from build123d import *

# Parameters (mm, degrees)
SKETCH2_W           = 32.5
SKETCH2_H           = 32.5
SKETCH2_R           = 1
BOSS_EXTRUDE1_DEPTH = 1.5
SKETCH4_W           = 13
SKETCH4_H           = 13
BOSS_EXTRUDE2_DEPTH = 4
SKETCH6_W           = 10
SKETCH6_H           = 4.75
BOSS_EXTRUDE3_DEPTH = 6


with BuildPart() as part:
    # Sketch2 → Boss-Extrude1 (new body)
    with BuildSketch(Plane.XY):
        Rectangle(SKETCH2_W, SKETCH2_H)
        with Locations((13.875, 13.875)):
            Circle(SKETCH2_R, mode=Mode.SUBTRACT)
        with Locations((13.875, -13.875)):
            Circle(SKETCH2_R, mode=Mode.SUBTRACT)
        with Locations((-13.875, -13.875)):
            Circle(SKETCH2_R, mode=Mode.SUBTRACT)
        with Locations((-13.875, 13.875)):
            Circle(SKETCH2_R, mode=Mode.SUBTRACT)
    extrude(amount=BOSS_EXTRUDE1_DEPTH)

    # Sketch4 → Boss-Extrude2 (add)
    with BuildSketch(Plane.XY.offset(1.5)):
        Rectangle(SKETCH4_W, SKETCH4_H)
        with BuildLine():
            Line((8.925, -1.85), (-8.925, -1.85))
            ThreePointArc((-8.925, -1.85), (-10.775, 0), (-8.925, 1.85))
            Line((-8.925, 1.85), (8.925, 1.85))
            ThreePointArc((8.925, 1.85), (10.775, 0), (8.925, -1.85))
        make_face()
    extrude(amount=BOSS_EXTRUDE2_DEPTH)

    # Sketch5 → Revolve1 (revolve)
    with BuildSketch(Plane(origin=(0, 0, 0), x_dir=(1, 0, 0), z_dir=(0, 1, 0)), mode=Mode.PRIVATE) as revolve1_sk:
        Polygon((0, -5.5), (6.5, -5.5), (6.5, -13.4), (5.65, -13.4), (5.65, -18.4), (8.5, -18.4), (8.5, -22.9), (0, -22.9), align=None)
    revolve(revolve1_sk.sketch.rotate(Axis((0, 0, 0), (0, 0, 1)), 180), axis=Axis((0, 0, 0), (0, 0, 1)))

    # Sketch6 → Boss-Extrude3 (add)
    with BuildSketch(Plane(origin=(0, 0, 0), x_dir=(-1, 0, 0), z_dir=(0, 0, -1))):
        with Locations((0, -13.875)):
            Rectangle(SKETCH6_W, SKETCH6_H)
    extrude(amount=BOSS_EXTRUDE3_DEPTH)


solid = part.part
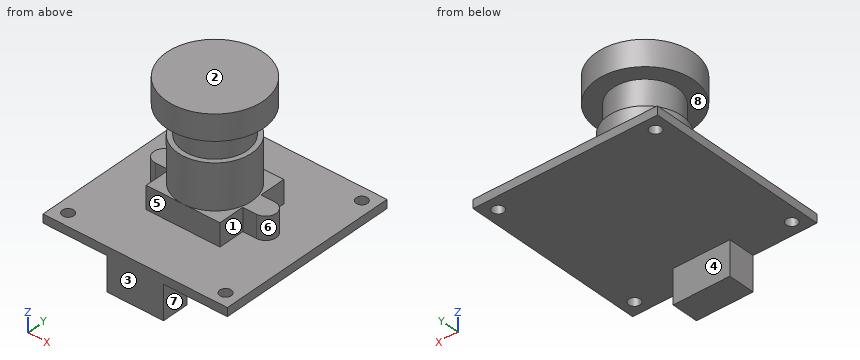
Can you work these out from the model? Positions are in its coordinate system, mm. Face numbers are marked on the shaded views. A direction names the side the tool comes from. Give positions to 0.01 mm unless a question says otherwise; leave off trailing zeros. Loops run counter-clockwise (first coordinate to the right, second up) from the corner with the lowest first, then second, coordinate; pieces in that order, holes last. Notation, with made-up numbers: (53, 80.25) - (92, 80.25) arc R18 ccw to (92, 90.25) - close; hole circle Ø8 at (12, 36.5). An arc over 180 degrees is marked (long way). Return JSON: item names as keys, results as strings.
1. We'd pull the mould along Z, two halves only. Please class the marked faces 1, 2 and 3: +Z half, -Z half, draft (parallel to the pull), parting line (faces both ways), or undercut.
Output values:
{"face 1": "undercut", "face 2": "+Z half", "face 3": "draft"}
2. I want a section at C-C on x = -3. Please give me the cut outline in (y, z).
Output values:
{"outline": "(-16.25, -6) - (-11.5, -6) - (-11.5, 0) - (16.25, 0) - (16.25, 1.5) - (6.5, 1.5) - (6.5, 5.5) - (5.77, 5.5) - (5.77, 13.4) - (4.79, 13.4) - (4.79, 18.4) - (7.95, 18.4) - (7.95, 22.9) - (-7.95, 22.9) - (-7.95, 18.4) - (-4.79, 18.4) - (-4.79, 13.4) - (-5.77, 13.4) - (-5.77, 5.5) - (-6.5, 5.5) - (-6.5, 1.5) - (-16.25, 1.5) - close"}
3. If I drill on line 1 (Z direction, x = 5, y = 6); line 2 (Y direction, x = 0, z = 20); line 3 (Z direction, x = 10, y = -13), over which ranges is the centre line in solid material (lowest first)?
Output values:
{"line 1": "z = 0 to 5.5, 18.4 to 22.9", "line 2": "y = -8.5 to 8.5", "line 3": "z = 0 to 1.5"}
4. I want a section at A-A on y = -12. Please give me the cut outline in (x, z), and give its area (3 significant figures).
Output values:
{"outline": "(-16.25, 0) - (-5, 0) - (-5, -6) - (5, -6) - (5, 0) - (16.25, 0) - (16.25, 1.5) - (-16.25, 1.5) - close", "area": "109 mm²"}
5. I want a section at D-D on y = 0. Please give me the cut outline in (x, z) (3 decimals), and give its area (3 significant figures).
Output values:
{"outline": "(-16.25, 0) - (16.25, 0) - (16.25, 1.5) - (10.775, 1.5) - (10.775, 5.5) - (6.5, 5.5) - (6.5, 13.4) - (5.65, 13.4) - (5.65, 18.4) - (8.5, 18.4) - (8.5, 22.9) - (-8.5, 22.9) - (-8.5, 18.4) - (-5.65, 18.4) - (-5.65, 13.4) - (-6.5, 13.4) - (-6.5, 5.5) - (-10.775, 5.5) - (-10.775, 1.5) - (-16.25, 1.5) - close", "area": "371 mm²"}
6. I want a section at B-B on z = -1.75. Please give me the cut outline in (x, y).
Output values:
{"outline": "(-5, -16.25) - (5, -16.25) - (5, -11.5) - (-5, -11.5) - close"}
7. For the marked faces 4, 5, 6, 7 and 8, which set-ups out of +Z, -Z, +X, -X, +Y, -Y let a thin tool reach every point of the face, with its end or its side?
Output values:
{"face 4": "-Z, +X, -X, +Y", "face 5": "+X, -X, -Y", "face 6": "+Z, +X", "face 7": "-Z, +X, +Y, -Y", "face 8": "none"}
8. I'm going to push flat-ended pins straight in: pin 1 Ø1.2 at (x, y) = (-13.875, 13.875) entering from -Z; pin 2 Ø4 at (x, z) = (7, 18.5) entering from +Y; pin 3 Ø1.9 at (x, z) = (-7, 3) entering from +Y; pin 4 Ø1.2 at (x, z) = (-8.5, 3) entering from -Y. Where does each tip first touch, or does it pass through?
Output values:
{"pin 1": "passes through", "pin 2": "stops at y = 6.87", "pin 3": "stops at y = 6.5", "pin 4": "stops at y = -1.85"}
